Here's how the part is built. I have some questions about the finished solid (model axes, mm). Coordinates: 2 decimals unless noted, no trailing zeros. Loops run counter-clockwise (first coordinate to the right, second up) from the corner with the lowest first, then second, coordinate; pieces in that order, holes last. Notation, with made-up numbers: (56.5, -23) -> (65.5, -23) arc R26 ccw to (65.5, 13) -> close; hole circle Ø5 at (64.25, 61.25). An arc over 180 degrees is marked (long way). Answer as a JSON object with one key per item and string values. Group by question number.
Q1. I want a section at B-B on y = 24.5. Write out the boundary of the cut face in (x, z).
Q2. I want a section at C-C on z = 1.65. Count the separate pieces of the cut face and the enclosed holes in it, then the cut area to 3 significant figures.
Q3. I need wall thicknesses on line 1 (X direction, y = 54, z = 0.7); line 2 (Y direction, x = -120.8, z = 1.75); line 3 (X direction, y = 42.5, z = 0.6). Which ranges of each line are inside material? Lowest first, please.
Q4. I want a section at A-A on y = -51. Write out the boundary of the cut face in (x, z).
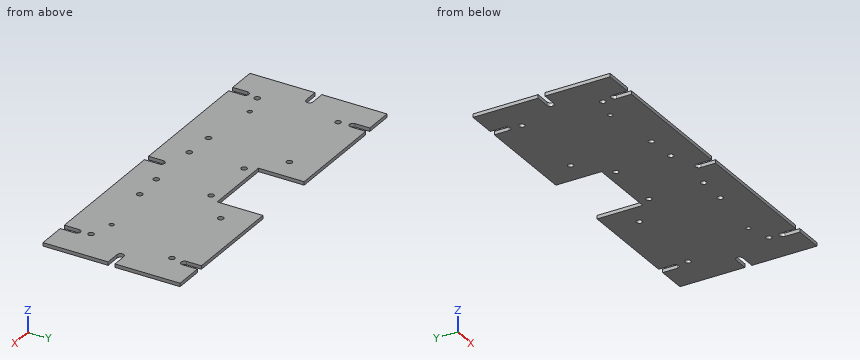
```python
from build123d import *

# Parameters (mm, degrees)
SKETCH1_W           = 301
SKETCH1_H           = 120
BOSS_EXTRUDE1_DEPTH = 3
SKETCH2_W           = 60
SKETCH2_H           = 40
CUT_EXTRUDE1_DEPTH  = 3
CUT_EXTRUDE2_DEPTH  = 10
SKETCH5_R           = 2.5
CUT_EXTRUDE3_DEPTH  = 10
SKETCH6_R           = 2.5
CUT_EXTRUDE4_DEPTH  = 10
SKETCH7_R           = 2
CUT_EXTRUDE5_DEPTH  = 10


with BuildPart() as part:
    # Sketch1 → Boss-Extrude1 (new body)
    with BuildSketch(Plane.XY):
        Rectangle(SKETCH1_W, SKETCH1_H)
    extrude(amount=BOSS_EXTRUDE1_DEPTH)

    # Sketch2 → Cut-Extrude1 (cut)
    with BuildSketch(Plane.XY.offset(3)):
        with Locations((0, 40)):
            Rectangle(SKETCH2_W, SKETCH2_H)
    extrude(amount=-CUT_EXTRUDE1_DEPTH, mode=Mode.SUBTRACT)

    # Sketch4 → Cut-Extrude2 (cut)
    with BuildSketch(Plane.XY.offset(3)):
        with BuildLine():
            Line((-125.5, -47), (-125.5, -60))
            Line((-125.5, -60), (-119.5, -60))
            Line((-119.5, -60), (-119.5, -47))
            ThreePointArc((-119.5, -47), (-122.5, -44), (-125.5, -47))
        make_face()
        with BuildLine():
            Line((-150.5, 3), (-150.5, -3))
            Line((-150.5, -3), (-137.5, -3))
            ThreePointArc((-137.5, -3), (-134.5, 0), (-137.5, 3))
            Line((-137.5, 3), (-150.5, 3))
        make_face()
        with BuildLine():
            Line((119.5, -47), (119.5, -60))
            Line((119.5, -60), (125.5, -60))
            Line((125.5, -60), (125.5, -47))
            ThreePointArc((125.5, -47), (122.5, -44), (119.5, -47))
        make_face()
        with BuildLine():
            Line((137.5, -3), (150.5, -3))
            Line((150.5, -3), (150.5, 3))
            Line((150.5, 3), (137.5, 3))
            ThreePointArc((137.5, 3), (134.5, 0), (137.5, -3))
        make_face()
        with BuildLine():
            Line((125.5, 47), (125.5, 60))
            Line((125.5, 60), (119.5, 60))
            Line((119.5, 60), (119.5, 47))
            ThreePointArc((119.5, 47), (122.5, 44), (125.5, 47))
        make_face()
        with BuildLine():
            Line((-119.5, 47), (-119.5, 60))
            Line((-119.5, 60), (-125.5, 60))
            Line((-125.5, 60), (-125.5, 47))
            ThreePointArc((-125.5, 47), (-122.5, 44), (-119.5, 47))
        make_face()
        with BuildLine():
            Line((3, -47), (3, -60))
            Line((3, -60), (-3, -60))
            Line((-3, -60), (-3, -47))
            ThreePointArc((-3, -47), (0, -44), (3, -47))
        make_face()
    extrude(amount=-CUT_EXTRUDE2_DEPTH, mode=Mode.SUBTRACT)

    # Sketch5 → Cut-Extrude3 (cut)
    with BuildSketch(Plane.XY.offset(3)):
        with Locations((120.8, 35)):
            Circle(SKETCH5_R)
        with Locations((120.8, -35.8)):
            Circle(SKETCH5_R)
        with Locations((50, -35.8)):
            Circle(SKETCH5_R)
        with Locations((50, 35)):
            Circle(SKETCH5_R)
    cut_extrude3 = extrude(amount=-CUT_EXTRUDE3_DEPTH, mode=Mode.SUBTRACT)

    # Mirror1: Cut-Extrude3 across plane
    add(cut_extrude3.mirror(Plane.ZY), mode=Mode.SUBTRACT)

    # Sketch6 → Cut-Extrude4 (cut)
    with BuildSketch(Plane.XY.offset(3)):
        with Locations((24, 11)):
            Circle(SKETCH6_R)
        with Locations((-24, 11)):
            Circle(SKETCH6_R)
        with Locations((-24, -37)):
            Circle(SKETCH6_R)
        with Locations((24, -37)):
            Circle(SKETCH6_R)
    extrude(amount=-CUT_EXTRUDE4_DEPTH, mode=Mode.SUBTRACT)

    # Sketch7 → Cut-Extrude5 (cut)
    with BuildSketch(Plane.XY.offset(3)):
        with Locations((-100.5, -30)):
            Circle(SKETCH7_R)
        with Locations((100.5, -30)):
            Circle(SKETCH7_R)
    extrude(amount=-CUT_EXTRUDE5_DEPTH, mode=Mode.SUBTRACT)


solid = part.part
```
Result set:
{
 "1": {"outline": "(-150.5, 0) -> (-30, 0) -> (-30, 3) -> (-150.5, 3) -> close; (30, 0) -> (150.5, 0) -> (150.5, 3) -> (30, 3) -> close"},
 "2": {"separate pieces": "1", "enclosed holes": "14", "area": "32,800 mm²"},
 "3": {"line 1": "x = -150.5 to -125.5, -119.5 to -30, 30 to 119.5, 125.5 to 150.5", "line 2": "y = -44.53 to -38.3, -33.3 to 32.5, 37.5 to 44.53", "line 3": "x = -150.5 to -30, 30 to 150.5"},
 "4": {"outline": "(-150.5, 0) -> (-125.5, 0) -> (-125.5, 3) -> (-150.5, 3) -> close; (-119.5, 0) -> (-3, 0) -> (-3, 3) -> (-119.5, 3) -> close; (3, 0) -> (119.5, 0) -> (119.5, 3) -> (3, 3) -> close; (125.5, 0) -> (150.5, 0) -> (150.5, 3) -> (125.5, 3) -> close"}
}
